```python
from build123d import *

# Parameters (mm, degrees)
SKETCH1_R           = 30
BOSS_EXTRUDE1_DEPTH = 32
CUT_EXTRUDE1_DEPTH  = 64
BOSS_EXTRUDE2_DEPTH = 20
SKETCH4_R           = 7.5
SKETCH4_R_2         = 2.5
CUT_EXTRUDE2_DEPTH  = 64
CIRPATTERN1_COUNT   = 8
BOSS_EXTRUDE3_DEPTH = 13
SKETCH6_R           = 7.5
CUT_EXTRUDE3_DEPTH  = 64


with BuildPart() as part:
    # Sketch1 → Boss-Extrude1 (new, symmetric)
    with BuildSketch(Plane(origin=(0, 0, 0), x_dir=(0, 0, -1), z_dir=(1, 0, 0))):
        with BuildLine():
            Line((0, 0), (11.471528727, -16.383040886))
            Line((11.471528727, -16.383040886), (119.001754001, 58.910433436))
            ThreePointArc((119.001754001, 58.910433436), (157.019843873, 51.167795707), (183.721445355, 79.316473737))
            Line((183.721445355, 79.316473737), (262.991611893, 79.316473737))
            Line((262.991611893, 79.316473737), (262.991611893, 82.816473737))
            Line((262.991611893, 82.816473737), (300.991611893, 82.816473737))
            Line((300.991611893, 82.816473737), (300.991611893, 95.816473737))
            Line((300.991611893, 95.816473737), (262.991611893, 95.816473737))
            Line((262.991611893, 95.816473737), (262.991611893, 99.316473737))
            Line((262.991611893, 99.316473737), (183.721445355, 99.316473737))
            ThreePointArc((183.721445355, 99.316473737), (132.963379912, 127.465151767), (107.530225274, 75.293474322))
            Line((107.530225274, 75.293474322), (0, 0))
        make_face()
        with Locations((144.991611893, 89.316473737)):
            Circle(SKETCH1_R, mode=Mode.SUBTRACT)
    extrude(amount=BOSS_EXTRUDE1_DEPTH, both=True)

    # Sketch2 → Cut-Extrude1 (cut)
    with BuildSketch(Plane(origin=(0, 0, 0), x_dir=(1, 0, 0), z_dir=(0, 0.8191520442889949, 0.5735764363510418))):
        with BuildLine():
            Line((25, -20), (-25, -20))
            ThreePointArc((-25, -20), (-45, 0), (-25, 20))
            Line((-25, 20), (25, 20))
            ThreePointArc((25, 20), (45, 0), (25, -20))
        make_face()
    extrude(amount=-CUT_EXTRUDE1_DEPTH, mode=Mode.SUBTRACT)

    # Sketch3 → Boss-Extrude2 (add)
    with BuildSketch(Plane(origin=(0, 0, 0), x_dir=(1, 0, 0), z_dir=(0, 0.8191520442889949, 0.5735764363510418))):
        with BuildLine():
            Line((25, -20), (-25, -20))
            ThreePointArc((-25, -20), (-45, 0), (-25, 20))
            Line((-25, 20), (25, 20))
            ThreePointArc((25, 20), (45, 0), (25, -20))
        make_face()
        with BuildLine():
            Line((25, -7.5), (-25, -7.5))
            ThreePointArc((-25, -7.5), (-32.5, 0), (-25, 7.5))
            Line((-25, 7.5), (25, 7.5))
            ThreePointArc((25, 7.5), (32.5, 0), (25, -7.5))
        make_face(mode=Mode.SUBTRACT)
    extrude(amount=-BOSS_EXTRUDE2_DEPTH)

    # Sketch4 → Cut-Extrude2 (cut)
    with BuildSketch(Plane(origin=(0, 99.316473737, 0), x_dir=(1, 0, 0), z_dir=(0, 1, 0))):
        with Locations(Location((0, 223.371445355, 0), (0, 0, 270))):
            Circle(SKETCH4_R)
        with Locations(Location((0, 243.181528624, 0), (0, 0, 270))):
            Circle(SKETCH4_R_2)
    cut_extrude2 = extrude(amount=-CUT_EXTRUDE2_DEPTH, mode=Mode.SUBTRACT)

    # CirPattern1: Cut-Extrude2 ×8 about axis
    cirpattern1_axis = Axis((0, 0, -223.371445355), (0, 1, 0))
    for i in range(1, CIRPATTERN1_COUNT):
        add(cut_extrude2.rotate(cirpattern1_axis, i * 360 / CIRPATTERN1_COUNT), mode=Mode.SUBTRACT)

    # Sketch5 → Boss-Extrude3 (add)
    with BuildSketch(Plane(origin=(0, 95.816473737, 0), x_dir=(1, 0, 0), z_dir=(0, 1, 0))):
        with BuildLine():
            Line((-32, 300.991611893), (32, 300.991611893))
            ThreePointArc((32, 300.991611893), (0, 332.991611893), (-32, 300.991611893))
        make_face()
    extrude(amount=-BOSS_EXTRUDE3_DEPTH)

    # Sketch6 → Cut-Extrude3 (cut)
    with BuildSketch(Plane(origin=(0, 95.816473737, 0), x_dir=(1, 0, 0), z_dir=(0, 1, 0))):
        with Locations(Location((0, 300.991611893, 0), (0, 0, 270))):
            Circle(SKETCH6_R)
    extrude(amount=-CUT_EXTRUDE3_DEPTH, mode=Mode.SUBTRACT)


solid = part.part
```
Here's how the part is built. I have some questions about the finished solid (model axes, mm). A direction names the side the tool comes from. Give positions to 0.01 mm unless a question says otherwise; leave off trailing zeros. Write each loop counter-clockwise with the first axis right and the second up, starting at its lowest first coordinate (ties: lowest second). Pieces come first, ordered by that corner, then holes. Notation, with made-up numbers: (-38.5, -32.5) -> (-25.5, -32.5) arc R14 cw to (-25.5, -7.5) -> close; hole circle Ø11 at (7.25, 34.25). An arc over 180 degrees is marked (long way). Use one line per item in the form item = value.
1) We'd pull the mould along Z, two halves only. Please class faces 1 (the face through (0.448, 127.729, -133.834)), 2 (the face through (-0.35, -3.775, -11.799)), 3 (the face through (-32, 57, -147)), 4 (the face through (0.704, 89.407, -332.984)): +Z half, -Z half, draft (parallel to the pull), parting line (faces both ways), or undercut.
Verdict:
face_1 = parting line
face_2 = undercut
face_3 = draft
face_4 = -Z half
2) Suppose I cut it at A-A (z = -126). Please give me the cut outline in (x, y), and give its area (3 significant figures).
Verdict:
outline = (-32, 54.11) -> (32, 54.11) -> (32, 66.09) -> (-32, 66.09) -> close; (-32, 112.54) -> (32, 112.54) -> (32, 124.52) -> (-32, 124.52) -> close
area = 1,530 mm2
3) I'm going to push flat-ended pins straight in: pin 1 (17 mm diameter, centred on x = 0, z = -223.37, fed in from -Y); pin 2 (19 mm diameter, centred on x = 15, z = -285, fed in from -Y); pin 3 (3 mm diameter, centred on x = 32, z = -163, fed in from +Y). Where does each tip first touch, or does it pass through?
Verdict:
pin_1 = 79.32
pin_2 = 82.82
pin_3 = 125.75
4) On a 3-axis mill with a long thin cutter (end or side, diameter ignored), from which of +Z, -Z, +X, -X, +Y, -Y can I reach the whole of each face in a straight line? I mean faces 5 (the face through (8, 99.316, -224)), 6 (the face through (0.35, -12.379, 0.488)), 7 (the face through (-2.873, 89.456, -216.443)), 8 (the face through (8, 79.316, -223)), 9 (the face through (-32.5, -8.17, -5.52)). Say none if no direction works.
Verdict:
face_5 = -Z, +X, -X, +Y
face_6 = +Y
face_7 = +Y, -Y
face_8 = -Z, +X, -X, -Y
face_9 = none
5) Suppose I cut it at B-B (z = -39). Please give me the cut outline in (x, y), and give its area (3 significant figures).
Verdict:
outline = (-32, 2.89) -> (32, 2.89) -> (32, 27.31) -> (-32, 27.31) -> close
area = 1,560 mm2
6) If I drill on L1, parallel to X at y = 83, z = -300.5; L2, parallel to X at y = -1, z = -2; L3, parallel to Y at x = 16.5, z = -305, over which ranges is the centre line in solid material (lowest first)? Write a range as [from, to].
Verdict:
L1 = [-32, -7.48], [7.48, 32]
L2 = [-44.97, -32.42], [32.42, 44.97]
L3 = [82.82, 95.82]
